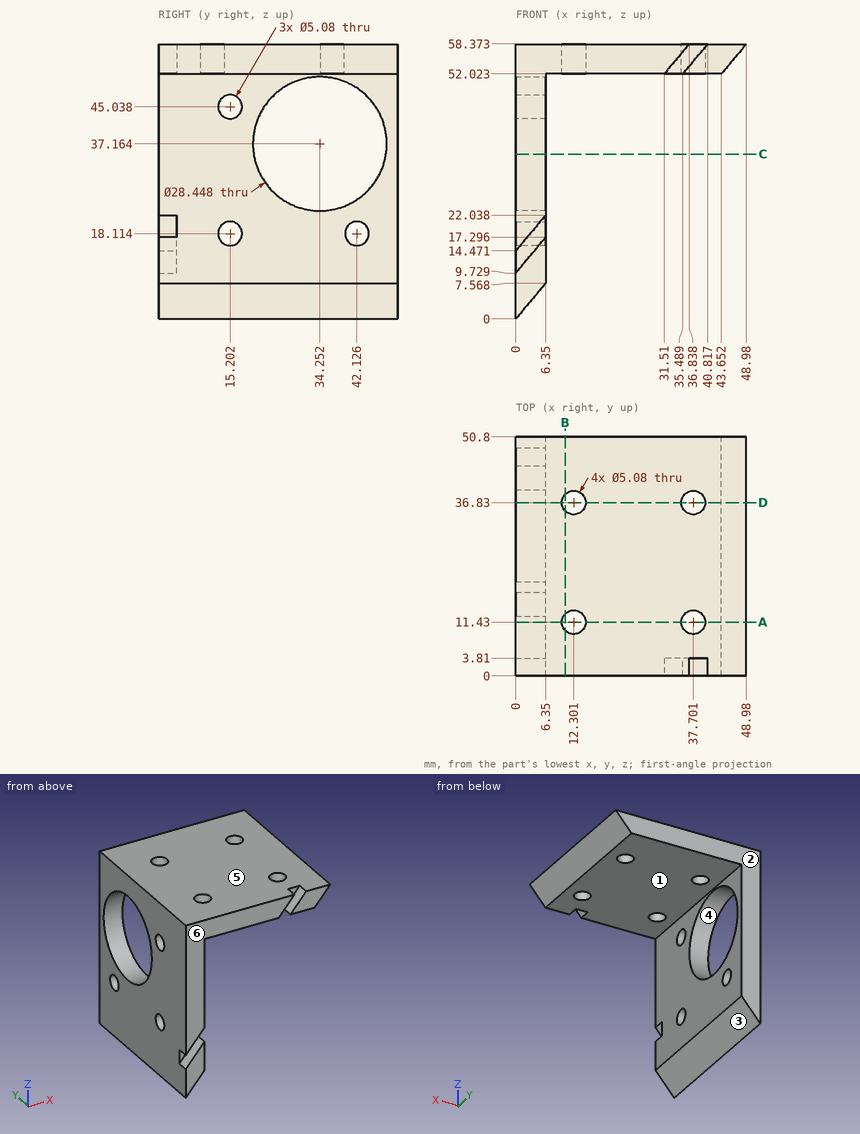
Answer from the drawing. Dimensions are ordinates in mm from the lowest x, y and z of the part. A direction names the side the tool comes from. Give positions to 0.01 mm unless a question says otherwise; leave off trailing zeros. Order: outer loops, then holes, each group sorted by start corner. A loop starts at its lowest first (then second) coordinate and runs counter-clockwise, first axis right, second up. Notation, with made-up numbers: (19, -28) - (54, -28) arc R16 ccw to (54, -19) - close; hole circle Ø2 at (51.25, 53.5). An arc over 180 degrees is marked (long way). One line per item, written item: value. Start each with the question number.
1) The mould has two halves that part along Z. Classify the marked faces 3, 4, 5 and 6: released by +Z, released by -Z, zero draft, split by the parting line, or undercut.
2) A cutting plane is placed at D-D on y = 36.83. State how many separate pieces and enclosed holes the cut face has, then the cut area to 3 significant figures.
3) Find the intervals of material crossed by L1, parallel to X at y = 40, z = 51; L2, parallel to Z at x = 8, y = 29; L3, parallel to Z at x = 3.5, y = 32 (1 decimal), in increasing order.
4) A cutting plane is placed at C-C on z = 35. Give the vertices of the cut face in (x, y), then the cut area to 3 significant figures.
5) A tool of negligible diameter and unlimited length cuts with its end or side. For the marked faces 1 and 2, from which of +Z, -Z, +X, -X, +Y, -Y can it reach the whole face along a straight path? Write none if from no direction.
6) Given pin 1 Ø4.5 at (x, y) = (12.3, 36.83) entering from +Z; pin 2 Ø12 at (x, y) = (35.5, 32.5) entering from -Z; pin 3 Ø22 at (y, z) = (36, 24.5) entering from +X, each flat-ended and moving along its own axis, determine where each tip first touches the part or whether it passes through.
7) A cutting plane is placed at B-B on x = 10.5. Give the vertices of the cut face in (y, z).
8) A cutting plane is placed at A-A on y = 11.43. Give the vertices of the cut face in (x, z).
Answer sheet:
1. face 3: released by -Z
1. face 4: undercut
1. face 5: released by +Z
1. face 6: zero draft
2. separate pieces: 4
2. enclosed holes: 0
2. area: 358 mm2
3. L1: x = 0 to 6.35
3. L2: z = 52.02 to 58.37
3. L3: z = 4.2 to 23.1, 51.2 to 58.4
4. outline: (0, 0) - (6.35, 0) - (6.35, 20.19) - (0, 20.19) - close; (0, 48.31) - (6.35, 48.31) - (6.35, 50.8) - (0, 50.8) - close
4. area: 144 mm2
5. face 1: -Z, +X, +Y, -Y
5. face 2: +Z, -Z, +X, -X, +Y
6. pin 1: passes through
6. pin 2: stops at z = 52.02
6. pin 3: stops at x = 6.35
7. outline: (0, 52.02) - (9.64, 52.02) - (9.64, 58.37) - (0, 58.37) - close; (13.22, 52.02) - (35.04, 52.02) - (35.04, 58.37) - (13.22, 58.37) - close; (38.62, 52.02) - (50.8, 52.02) - (50.8, 58.37) - (38.62, 58.37) - close
8. outline: (0, 0) - (6.35, 7.57) - (6.35, 52.02) - (9.76, 52.02) - (9.76, 58.37) - (0, 58.37) - close; (14.84, 52.02) - (35.16, 52.02) - (35.16, 58.37) - (14.84, 58.37) - close; (40.24, 52.02) - (43.65, 52.02) - (48.98, 58.37) - (40.24, 58.37) - close
